Autodesk Inventor part; units mm, degrees
ref_plane "Work Plane1" through (25, 0, 0) normal (0, 0.5, 0.866) x (1, 0, 0)
ref_plane "YZ Plane" through (0, 0, 0) normal (1, 0, 0) x (0, 1, 0)
ref_plane "XZ Plane" through (0, 0, 0) normal (0, 1, 0) x (-1, 0, 0)
sketch "Sketch1" plane through (0, 0, 0) normal (0, 0, 1) x (1, 0, 0)
  line L0 (1.0774, 0) -> (50, 0)
  line L1 (50, 0) -> (50, 2)
  line L2 (50, 2) -> (0, 2)
  line L3 (0, 2) -> (0, 3.5)
  line L4 (0, 3.5) -> (-2.8, 3.5)
  line L5 (-2.8, 3.5) -> (-2.8, 1.7321)
  line L6 (-2.8, 1.7321) -> (-1.2, 1.7321)
  line L7 (-1.2, 1.7321) -> (-0.7774, 1)
  line L8 (-13.36, 0) -> (60.56, 0)
  line L9 (0, -0.7) -> (0, 4.2)
  line L10 (-0.7774, 1) -> (0.5, 1)
  line L11 (0.5, 1) -> (1.0774, 0)
  line L12 (-2.8, 1.7321) -> (-2.8, 0) construction
  line L13 (-2.8, 3.1) -> (-2.4, 3.5)
  dimension "d0" = 2.8
  dimension "d1" = 1.6
  dimension "d2" = 60
  dimension "d3" = 4
  dimension "d4" = 3.4641
  dimension "d5" = 7
  dimension "d15" = 3.3
  dimension "d16" = 2
  dimension "d17" = 50
  dimension "d32" = 45
  dimension "d33" = 0.4
revolve "Body" add sketch "Sketch1" angle 360 about axis through (1.0774, 0, 0) along (1, 0, 0) contours L11 L10 L9 L2 L1 L0 | L10 L7 L6 L5 L13 L4 L3 L9 | L13 L5 L4
revolve "Chamfer2" cut sketch "Sketch1" angle 360 about axis through (-10, 0, 0) along (1, 0, 0) contours L13 L5 L4
sketch "Sketch2" plane through (-2.8, 0, 0) normal (-1, 0, 0) x (0, 0, 1)
  circle A0 centre (0, 0) radius 1.7321
  line L0 (0, -4.9) -> (0, 4.9)
  line L1 (-4.9, 0) -> (4.9, 0)
  line L2 (1.7321, 0) -> (0.866, -1.5)
  line L3 (0.866, -1.5) -> (-0.866, -1.5)
  line L4 (-0.866, -1.5) -> (-1.7321, 0)
  line L5 (-1.7321, 0) -> (-0.866, 1.5)
  line L6 (-0.866, 1.5) -> (0.866, 1.5)
  line L7 (0.866, 1.5) -> (1.7321, 0)
extrude "Slot" add sketch "Sketch2" against normal up to next contours L7 A0 | A0 L2 | L6 L0 A0 | A0 L0 L3 | L0 L6 A0 | A0 L3 L0 | L4 A0 | A0 L5
thread "Thread"
chamfer "Chamfer1" distance 0.4294 distance2 0.4294 1 edges at (50, -2, 0) measured on face at (50, -0.8158, 0.4805)
ref_plane "Work Plane1" through (25, 0, 0) normal (0, 0.5, 0.866) x (1, 0, 0)
equation "\"d0\" = KOH"
equation "\"d1\" = INTI"
equation "\"d3\" = GD"
equation "\"d4\" = 1.1547 * SW"
equation "\"d5\" = KOD"
equation "\"d15\" = INFT"
equation "\"d16\" = SDT"
equation "\"d17\" = NLG"
equation "\"d33\" = Cham"
equation "\"d7\" = GEL"
equation "\"d9\" = -0.5 * SPD + 0.5 * GD"
equation "\"d12\" = GUL"
equation "\"GD\" = NND"
equation "\"NLG\" = 50"
equation "\"GEL\" = 14"
equation "\"KOD\" = 7"
equation "\"KOH\" = 2.8"
equation "\"GUL\" = 0.61345 * PTC"
equation "\"SW\" = 3"
equation "\"INTI\" = 1.6"
equation "\"SPD\" = NND - 1.2269 * PTC"
equation "\"SDT\" = 2"
equation "\"INFT\" = 3.3"
equation "\"Cham\" = 0.4"
equation "\"TOA\" = 30deg"
equation "\"GD1\" = THREADDIA - 1.2269 * PTC"
equation "\"THREADDIA\" = 4"
equation "\"BDM\" = NND"
equation "\"FAWI\" = 45deg"
equation "\"RR\" = 0.1 * NND"
equation "\"PTC\" = 0.7"
equation "\"NND\" = 4"
equation "\"FAWI1\" = 45deg"
equation "\"GAL\" = 0.61345 * PTC"
equation "\"E0\" = 1.155 * SW"
properties part number "DIN 6912 - M4 x 50" material "Steel, Mild"
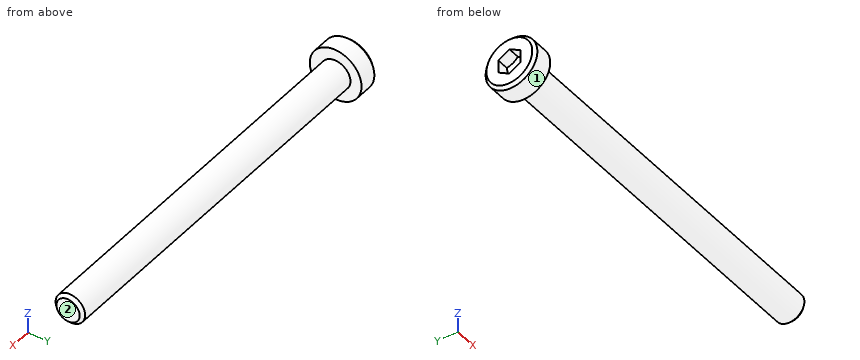
Work out the finished part from the listing and answer in its coordinate system (mm). Face numbers are marked on the shaded views. Coordinates: 2 decimals unless noted, no trailing zeros. Order: outer loops, then holes, each group sorted by start corner. A loop starts at its lowest first (then second) coordinate and runs counter-clockwise, first axis right, second up. Notation, with made-up numbers: (64.25, 53) - (71.25, 53) arc R16 ccw to (71.25, 78) - close; hole circle Ø3 at (15.5, 40.5). An arc over 180 degrees is marked (long way). Answer as a JSON object with one key per item and string values.
1. This flat-tipped pin is pushed along its axis until it touches: P1, Ø1, axis at x = 16.5, y = -0.5, coming from the -Z side. Where does it stop, or does it pass through?
Output values:
{"P1": "stops at z = -2"}
2. The mould has two halves that part along Y. Classify the marked faces 1 and 2: +Y half, -Y half, draft (parallel to the pull), parting line (faces both ways), or undercut.
Output values:
{"face 1": "parting line", "face 2": "draft"}
3. Consider line 1 (Z direction, x = -0.25, y = 0); line 2 (X direction, y = 0.5, z = 2.5); line 3 (Y direction, x = 25, z = 1). Determine where each line is inside the solid, lowest interval first.
Output values:
{"line 1": "z = -3.5 to -1, 1 to 3.5", "line 2": "x = -2.8 to 0", "line 3": "y = -1.73 to 1.73"}
4. Find section A-A on x = 8.5. Determine the outline of the cut face in (y, z), plus the area to 3 significant figures.
Output values:
{"outline": "circle Ø4 at (0, 0)", "area": "12.6 mm²"}
